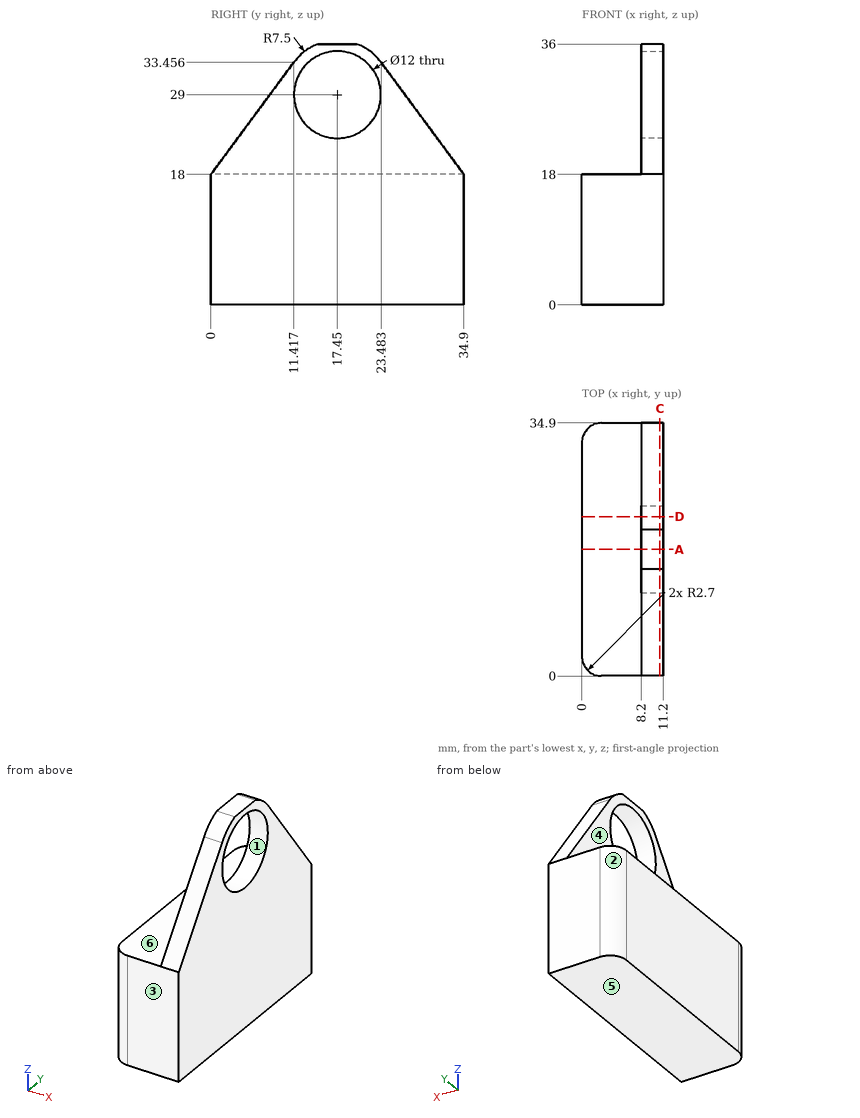
The drawing under review shows one solid part. Ordinate dimensions are in mm from its lowest x, y, z. A direction names the side the tool comes from. Round coordinates to 2 decimals unless told otherwise and drop trailing zeros. Loops run counter-clockwise (first coordinate to the right, second up) from the corner with the lowest first, then second, coordinate; pieces in that order, holes last. Notation, with made-up numbers: (75, 82.25) - (114, 82.25) arc R20 ccw to (114, 119.25) - close; hole circle Ø6 at (77, -26.75). An arc over 180 degrees is marked (long way). Put each result on its own line as item: value. Start each with the question number.
1. For the marked faces 5 and 6, list the 3-axis set-ups (+Z, -Z, +X, -X, +Y, -Y) from which the entire face can be reached by the end or side of a thin tool; tool diameter is ignored.
2. Consider section A-A on y = 17.45. State the section outline as (x, z) points.
3. Consider section C-C on x = 10.75. State the section outline as (y, z) points, plus the area to 3 significant figures.
4. Consider section D-D on y = 22. State the section outline as (x, z) points, plus the area to 3 significant figures.
5. Insertion check: P1, Ø14.5, axis at y = 16, z = 28, coming from the -X side; P2, Ø2.5, axis at x = 2.5, y = 22.5, coming from the +Z side. Each pin has a flat end and moves straight along its axis. Give the tip position at first contact, or say it passes through.
6. Mouldability with a two-part tool opening along Y and no side actions: class the marked faces 1, 2, 3 and 4 as +Y half, -Y half, draft (parallel to the pull), parting line (faces both ways), or undercut.
7. For probe 1 along X at (y, z) = (9.5, 30.5); probe 2 along Z at (x, y) = (8.25, 13) (1 decimal); probe 3 along Z at (x, y) = (5.5, 10.5), list the stretches that pass through material, from the lowest coordinate up. Write a range as [from, to].
Result sheet:
1. face 5: -Z, +X, -X, +Y, -Y
1. face 6: +Z, -X, +Y, -Y
2. outline: (0, 0) - (11.2, 0) - (11.2, 23) - (8.2, 23) - (8.2, 18) - (0, 18) - close; (8.2, 35) - (11.2, 35) - (11.2, 36) - (8.2, 36) - close
3. outline: (0, 0) - (34.9, 0) - (34.9, 18) - (23.48, 33.46) arc R7.5 ccw to (20.14, 36) - (14.76, 36) arc R7.5 ccw to (11.42, 33.46) - (0, 18) - close; hole circle Ø12 at (17.45, 29)
3. area: 902 mm^2
4. outline: (0, 0) - (11.2, 0) - (11.2, 25.09) - (8.2, 25.09) - (8.2, 18) - (0, 18) - close; (8.2, 32.91) - (11.2, 32.91) - (11.2, 34.96) - (8.2, 34.96) - close
4. area: 229 mm^2
5. P1: x = 8.2
5. P2: z = 18
6. face 1: undercut
6. face 2: +Y half
6. face 3: -Y half
6. face 4: draft
7. probe 1: [8.2, 11.2]
7. probe 2: [0, 25], [33, 35]
7. probe 3: [0, 18]
